from build123d import *

# Parameters (mm, degrees)
SKETCH1_W           = 12.7
SKETCH1_H           = 25.4
SKETCH1_W_2         = 6.35
SKETCH1_H_2         = 19.05
BOSS_EXTRUDE1_DEPTH = 431.8
CUT_EXTRUDE1_DEPTH  = 13.7
CUT_EXTRUDE2_DEPTH  = 13.7


with BuildPart() as part:
    # Sketch1 → Boss-Extrude1 (new body)
    with BuildSketch(Plane.XY):
        with Locations((6.35, 12.7)):
            Rectangle(SKETCH1_W, SKETCH1_H)
        with Locations((6.35, 12.7)):
            Rectangle(SKETCH1_W_2, SKETCH1_H_2, mode=Mode.SUBTRACT)
    extrude(amount=BOSS_EXTRUDE1_DEPTH)

    # Sketch2 → Cut-Extrude1 (cut, through all)
    with BuildSketch(Plane(origin=(12.7, 0, 0), x_dir=(0, 0, -1), z_dir=(1, 0, 0))):
        Polygon((-431.8, 25.4), (-401.275136185, 0), (-431.8, 0), align=None)
    extrude(amount=-CUT_EXTRUDE1_DEPTH, mode=Mode.SUBTRACT)

    # Sketch3 → Cut-Extrude2 (cut, through all)
    with BuildSketch(Plane(origin=(12.7, 0, 0), x_dir=(0, 0, -1), z_dir=(1, 0, 0))):
        Polygon((-21.13555703, 0), (0, 25.4), (0, 0), align=None)
    extrude(amount=-CUT_EXTRUDE2_DEPTH, mode=Mode.SUBTRACT)


solid = part.part
Could you check a few things on this model? Use its own coordinates, in mm. Give positions to 0.01 mm unless a question says otherwise; leave off trailing zeros. Order: outer loops, then holes, each group sorted by start corner. A loop starts at its lowest first (then second) coordinate and runs counter-clockwise, first axis right, second up. Notation, with made-up numbers: (-17, 66.5) - (3, 66.5) arc R18 cw to (3, 86.5) - close; hole circle Ø8 at (79.25, 56.25). An arc over 180 degrees is marked (long way). Return JSON: item names as keys, results as strings. Group by question number.
Q1. Please list where these lines run through material, in increasing order: line 1 along Y through (x, z) = (4.5, 80.5) (3 decimals); line 2 along X through (y, z) = (13.75, 197) (3 decimals); line 3 along Z through (x, y) = (1.75, 4.5). Write a range as [from, to].
Q2. Suppose I cut it at B-B, the plane z = 117.5. Please give me the cut outline in (x, y) (3 decimals).
Q3. Suppose I cut it at A-A, the plane y = 11.25. Please give me the cut outline in (x, z) (3 decimals), and give its area (3 significant figures).
Q4. Thinking about a two-plate mould opening in X: for faces 1 (the face through (9.525, 13, 212)), 2 (the face through (3.175, 13, 212)), 3 (the face through (10.67, 12.52, 10.72)), 4 (the face through (0, 13, 213)), which applies, pulls with the +X half, pulls with the -X half, needs draft (parallel to the pull), parting line crosses it, or undercut?
Resolved:
{
 "1": {"line 1": "y = [0, 3.175], [22.225, 25.4]", "line 2": "x = [0, 3.175], [9.525, 12.7]", "line 3": "z = [17.39, 406.68]"},
 "2": {"outline": "(0, 0) - (12.7, 0) - (12.7, 25.4) - (0, 25.4) - close; hole (3.175, 3.175) - (9.525, 3.175) - (9.525, 22.225) - (3.175, 22.225) - close"},
 "3": {"outline": "(0, 11.774) - (3.175, 11.774) - (3.175, 414.795) - (0, 414.795) - close; (9.525, 11.774) - (12.7, 11.774) - (12.7, 414.795) - (9.525, 414.795) - close", "area": "2,560 mm2"},
 "4": {"face 1": "undercut", "face 2": "undercut", "face 3": "needs draft", "face 4": "pulls with the -X half"}
}
